Work out the finished part from the listing and answer in its coordinate system (mm). Face numbers are marked on the shaded views. Round coordinates to 2 decimals unless told otherwise and drop trailing zeros. Loops run counter-clockwise (first coordinate to the right, second up) from the corner with the lowest first, then second, coordinate; pieces in that order, holes last. Notation, with made-up numbers: (-20.75, 41) - (-13.75, 41) arc R22 cw to (-13.75, 72) - close; hole circle Ø1 at (48.5, 19). An arc over 180 degrees is marked (long way). Return JSON: item names as keys, results as strings.
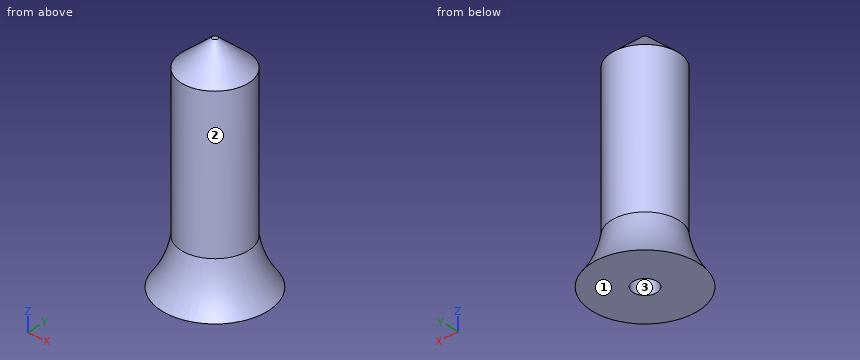
from build123d import *

# Parameters (mm, degrees)
F0_R     = 31.75
F0_R_2   = 11.43
F1_DEPTH = 185.71182
F4_R     = 31.75
F5_DEPTH = 25.4
F5_TAPER = 49


with BuildPart() as f1:
    # F0 (on Top) → F1 (new body)
    with BuildSketch(Plane.XY):
        Circle(F0_R)
        Circle(F0_R_2, mode=Mode.SUBTRACT)
    extrude(amount=F1_DEPTH)

    # F2 (on Front) → F3 (revolve)
    with BuildSketch(Plane.XZ):
        with BuildLine():
            ThreePointArc((-30.6478571147, 58.2644540342), (-35.6754691099, 27.5302272186), (-50.2341836691, 0))
            Line((-50.2341836691, 0), (-30.6478571147, 0))
            Line((-30.6478571147, 0), (-30.6478571147, 58.2644540342))
        make_face()
    revolve(axis=Axis((0, 0, 38.0581654608), (0, 0, -1)))

    # F4 (on face) → F5 (join)
    with BuildSketch(Plane.XY.offset(185.71182)):
        Circle(F4_R)
    extrude(amount=F5_DEPTH, taper=F5_TAPER)


solid = f1.part
1) Find the intervals of material crossed by L1, parallel to Y at x = -1, z = 99.5; L2, parallel to X at y = -0.5, z = 111; L3, parallel to X at y = 1.5, z = 171, in increasing order.
Verdict:
{"L1": "y = -31.73 to -11.39, 11.39 to 31.73", "L2": "x = -31.75 to -11.42, 11.42 to 31.75", "L3": "x = -31.71 to -11.33, 11.33 to 31.71"}
2) Flat-ended cylindrical pins translate along their axes: pin 1 (10 mm diameter, centred on x = -21, z = 116, fed in from -Y); pin 2 (3 mm diameter, centred on y = -26, z = 165, fed in from -X); pin 3 (11.5 mm diameter, centred on x = -1.5, y = 3, fed in from -Z). Find the tip coordinate at first contact, or state that the pin passes through.
Verdict:
{"pin 1": "stops at y = -27.42", "pin 2": "stops at x = -20.19", "pin 3": "stops at z = 185.71"}
3) Section C-C (z = 167.5) is taken. Give the vertices of the cut face in (x, y).
Verdict:
{"outline": "circle Ø63.5 at (0, 0); hole circle Ø22.86 at (0, 0)"}
4) Section A-A (y = 0) is taken. Give the vertices of the cut face in (x, z), and give its area (3 significant figures).
Verdict:
{"outline": "(-50.23, 0) - (-11.43, 0) - (-11.43, 185.71) - (11.43, 185.71) - (11.43, 0) - (50.23, 0) arc R96.45 cw to (31.75, 43.72) - (31.75, 185.71) - (2.53, 211.11) - (-2.53, 211.11) - (-31.75, 185.71) - (-31.75, 43.72) arc R96.45 cw to start", "area": "9,040 mm2"}
5) Section D-D (z = 36) is taken. Give the vertices of the cut face in (x, y).
Verdict:
{"outline": "circle Ø66.51 at (0, 0); hole circle Ø22.86 at (0, 0)"}
6) Determine the mould class of the marked faces 1, 2 and 3 for opening direction X: pulls with the +X half, pulls with the -X half, needs draft (parallel to the pull), parting line crosses it, or undercut.
Verdict:
{"face 1": "needs draft", "face 2": "parting line crosses it", "face 3": "undercut"}
